```python
from build123d import *

# Parameters (mm, degrees)
F1_DEPTH = 20
F3_D     = 42
F3_DEPTH = 50
F3_TIP   = 12.6180729996
F4_DEPTH = 25


with BuildPart() as f1:
    # F0 (on Front) → F1 (new body)
    with BuildSketch(Plane.XZ):
        Polygon((-13.2030190676, 2.2544430345), (-37.2030190676, 26.2544430345), (-37.2030190676, -21.7455569655), align=None)
        Polygon((10.7969809324, 26.2544430345), (-37.2030190676, 26.2544430345), (-13.2030190676, 2.2544430345), align=None)
        Polygon((10.7969809324, -21.7455569655), (10.7969809324, 26.2544430345), (-13.2030190676, 2.2544430345), align=None)
        Polygon((-13.2030190676, 2.2544430345), (-37.2030190676, -21.7455569655), (10.7969809324, -21.7455569655), align=None)
    extrude(amount=F1_DEPTH)

    # F3
    with Locations(Plane(origin=(0, 0, 0), x_dir=(-1, 0, 0), z_dir=(0, 1, 0))):
        with Locations((13.2030190676, 2.2544430345)):
            Hole(F3_D / 2, depth=F3_DEPTH)
            with Locations((0, 0, -(F3_DEPTH + F3_TIP / 2))):  # 118° drill point
                Cone(0, F3_D / 2, F3_TIP, mode=Mode.SUBTRACT)

    # F2 (on face) → F4 (join)
    with BuildSketch(Plane(origin=(0, 0, 0), x_dir=(-1, 0, 0), z_dir=(0, 1, 0))):
        Polygon((-10.7969809324, -21.7455569655), (37.2030190676, -21.7455569655), (13.2030190676, 2.2544430345), align=None)
        Polygon((13.2030190676, 26.2544430345), (13.2030190676, 2.2544430345), (37.2030190676, 26.2544430345), align=None)
        Polygon((13.2030190676, 2.2544430345), (37.2030190676, -21.7455569655), (37.2030190676, 26.2544430345), align=None)
    extrude(amount=F4_DEPTH)


solid = f1.part
```
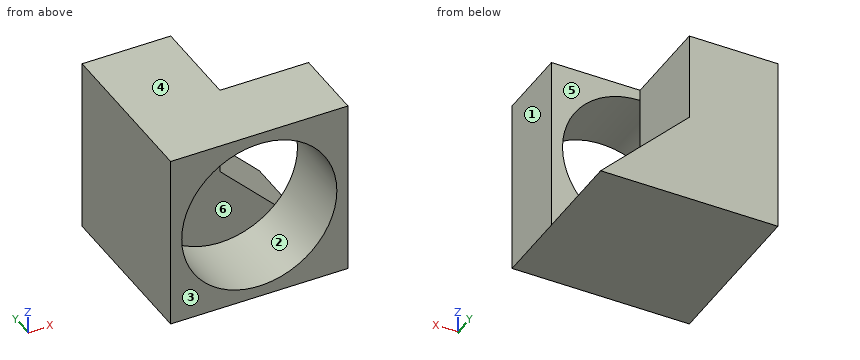
Input: part model. Units: mm. Frame: model coordinates. Face numbers are marked on the shaded views. A direction names the side the tool comes from. Give positions to 0.01 mm unless a question says otherwise; leave off trailing zeros. Loops run counter-clockwise (first coordinate to the right, second up) from the corner with the lowest first, then second, coordinate; pieces in that order, holes last. Notation, with made-up numbers: M 75.25,68.5 L 90.25,68.5 A12 cw 90.25,72.5 Z; hole C 37,15 d1. An arc over 180 degrees is marked long. Answer as CSV lines item,"result". Start each with the question number.
1. Reachability of the marked faces 4, 5 and 6 from +Z, -Z, +X, -X, +Y, -Y: full face, straight path, thin tool, end or side. Return the list, or none.
2. Section B-B on x = -4.5. Return loops of the section in (y, z), plus the area to 3 significant figures.
3. Section D-D on x = -14. Return loops of the section in (y, z).
4. Pull-direction query (X, two-part tool) for the marked faces 1, 2 and 3; classes: released by +X, released by -X, zero draft, split by the parting line, or undercut.
5. Line query: L1, parallel to X at y = 5.5, z = 19; L2, parallel to Y at x = -26.5, z = 7; L3, parallel to X at y = -14.5, z = 0. Output: solid intervals per line, ascending.
6. Pin query (flat end, axial travel): P1, Ø8, axis at x = -7.5, y = 19, coming from the +Z side; P2, Ø11, axis at x = -21, z = 0.5, coming from the -Y side; P3, Ø12, axis at x = -2, z = 15.5, coming from the +Y side; P4, Ø7, axis at x = 1, z = 9, coming from the +Y side. Return the tip coordinate at first contact, or that it passes through.
7. Section A-A on z = -10. Return loops of the section in (x, y).
8. Section C-C on y = -10. Return loops of the section in (x, z), plus the area to 3 significant figures.
Computed values:
1,face 4,"+Z, +X, -X, +Y, -Y"
1,face 5,"+Z, +X, +Y"
1,face 6,"-Y"
2,outline,"M -20,-21.75 L 25,-21.75 L 25,-6.45 L 0,-6.45 L 0,-16.86 L -20,-16.86 Z; M -20,21.37 L 0,21.37 L 0,26.25 L -20,26.25 Z"
2,area,"578 mm²"
3,outline,"M -20,-21.75 L 25,-21.75 L 25,26.25 L -20,26.25 L -20,23.24 L 0,23.24 L 0,-18.73 L -20,-18.73 Z"
4,face 1,"released by +X"
4,face 2,"undercut"
4,face 3,"zero draft"
5,L1,"x = -37.2 to -13.2"
5,L2,"y = 0 to 25"
5,L3,"x = -37.2 to -34.08, 7.68 to 10.8"
6,P1,"stops at z = 0.55"
6,P2,"stops at y = 0"
6,P3,"stops at y = 0"
6,P4,"passes through"
7,outline,"M -37.2,-20 L -30.26,-20 L -30.26,0 L -0.95,0 L -0.95,25 L -37.2,25 Z; M 3.85,-20 L 10.8,-20 L 10.8,0 L 3.85,0 Z"
8,outline,"M -37.2,-21.75 L 10.8,-21.75 L 10.8,26.25 L -37.2,26.25 Z; hole C -13.2,2.25 d42"
8,area,"919 mm²"
